CAD build for the part. Positions are in the model's coordinates, mm. A direction names the side the tool comes from. Give positions to 0.01 mm unless a question says otherwise; leave off trailing zeros. Write each loop counter-clockwise with the first axis right and the second up, starting at its lowest first coordinate (ties: lowest second). Pieces come first, ordered by that corner, then holes. Notation, with made-up numbers: (79, 18) - (105, 18) arc R15 cw to (105, 46) - close; hole circle Ø2 at (47, 79). An arc over 180 degrees is marked (long way). Put each result on its own line as item: value. Start each with the question number.
1. Wall check: line 1 (X direction, y = 1.7, z = 0); line 2 (Y direction, x = 0.9, z = 0); line 3 (Y direction, x = 1.3, z = 0). Give the ranges that are in metal, low to high.
2. Cut at B-B on z = 0. Give the number of separate pieces and of enclosed holes in the cut face, and give its area (3 significant figures).
3. Cut at A-A on x = 14.9. List the corners of the cut face in (y, z) (3 decimals).
4. Cut at D-D on x = 35. List the corners of the cut face in (y, z) (3 decimals), and give its area (3 significant figures).
5. Drop flat-ended pins along their axis: pin 1 (6 mm diameter, centred on x = 42.9, z = 0, fed in from -Y); pin 2 (8 mm diameter, centred on x = 18.5, z = 0, fed in from +Y) (3 decimals). Give the stop position or say it passes through.
6. Tool access for faces 5 (the flat face through (3.175, 28, 0)), 6 (the flat face through (14, 2, 7.9)): list every direction of +Z, -Z, +X, -X, +Y, -Y with a clear straight run to the whole face (end or side of a thin tool).
7. Cut at C-C on z = -5.25. List the corners of the cut face in (x, y) (3 decimals), and give its area (3 significant figures).
8. Mould opens along Y. For faces 1 (the cylindrical face through (1.1, 45.01, -1.34)), 2 (the cylindrical face through (1.1, 13.4, 2)), 3 (the flat face through (28, 0, 0)), 4 (the cylindrical face through (45.01, 1.1, 1.34)) say: +Y half, -Y half, draft (parallel to the pull), parting line (faces both ways), or undercut.
from build123d import *

# Parameters (mm, degrees)
FLANGE_BASE1_DEPTH    = 7.9
FILETE2_RADIUS        = 7.9
FILETE2_LENGTH        = 3.175
FILETE4_RADIUS        = 7.9
FILETE4_LENGTH        = 3.175
ESBO_O6_R             = 2.5
CORTE_EXTRUS_O1_DEPTH = 71.07988745
ESBO_O7_R             = 2.5
CORTE_EXTRUS_O2_DEPTH = 71.07988745
CHANFRO2_SIZE         = 1


# Sheet-metal steps are written as plain solids
with BuildPart() as part:
    # Esboço1 → Flange-base1 (new, symmetric)
    with BuildSketch(Plane.XY):
        with BuildLine():
            Line((50.8, 0), (4.175, 0))
            ThreePointArc((4.175, 0), (1.222829189, 1.222829189), (0, 4.175))
            Line((0, 4.175), (0, 50.8))
            Line((0, 50.8), (3.175, 50.8))
            Line((3.175, 50.8), (3.175, 4.175))
            ThreePointArc((3.175, 4.175), (3.467893219, 3.467893219), (4.175, 3.175))
            Line((4.175, 3.175), (50.8, 3.175))
            Line((50.8, 3.175), (50.8, 0))
        make_face()
    extrude(amount=FLANGE_BASE1_DEPTH, both=True)

    # Filete2: full round fillet: the end face becomes a half cylinder, R = half its width
    filete2_face = Plane((1.5875, 50.8, 0), x_dir=(1, 0, 0), z_dir=(0, 1, 0))  # on the end face: x along it, z out of the body
    filete2_slab = filete2_face.offset(-FILETE2_RADIUS / 2) * Box(FILETE2_LENGTH, 2 * FILETE2_RADIUS, FILETE2_RADIUS, mode=Mode.PRIVATE)  # the body's end, R deep
    filete2_round = Plane((1.5875, 42.9, 0), x_dir=(0, 1, 0), z_dir=(1, 0, 0)) * Cylinder(FILETE2_RADIUS, FILETE2_LENGTH, mode=Mode.PRIVATE)  # its axis R under the face
    add(filete2_slab - filete2_round, mode=Mode.SUBTRACT)

    # Filete4: full round fillet: the end face becomes a half cylinder, R = half its width
    filete4_face = Plane((50.8, 1.5875, 0), x_dir=(0, -1, 0), z_dir=(1, 0, 0))  # on the end face: x along it, z out of the body
    filete4_slab = filete4_face.offset(-FILETE4_RADIUS / 2) * Box(FILETE4_LENGTH, 2 * FILETE4_RADIUS, FILETE4_RADIUS, mode=Mode.PRIVATE)  # the body's end, R deep
    filete4_round = Plane((42.9, 1.5875, 0), x_dir=(1, 0, 0), z_dir=(0, -1, 0)) * Cylinder(FILETE4_RADIUS, FILETE4_LENGTH, mode=Mode.PRIVATE)  # its axis R under the face
    add(filete4_slab - filete4_round, mode=Mode.SUBTRACT)

    # Esboço6 → Corte-extrusão1 (cut, through all)
    with BuildSketch(Plane(origin=(0, 3.175, 0), x_dir=(1, 0, 0), z_dir=(0, 1, 0))):
        with Locations(Location((14.9, 0, 0), (0, 0, 270))):
            Circle(ESBO_O6_R)
        with Locations(Location((42.9, 0, 0), (0, 0, 270))):
            Circle(ESBO_O6_R)
    extrude(amount=-CORTE_EXTRUS_O1_DEPTH, mode=Mode.SUBTRACT)

    # Esboço7 → Corte-extrusão2 (cut, through all)
    with BuildSketch(Plane(origin=(3.175, 0, 0), x_dir=(0, 0, -1), z_dir=(1, 0, 0))):
        with Locations((0, 42.9)):
            Circle(ESBO_O7_R)
        with Locations((0, 14.9)):
            Circle(ESBO_O7_R)
    extrude(amount=-CORTE_EXTRUS_O2_DEPTH, mode=Mode.SUBTRACT)

    # Chanfro2
    chanfro2_edges = [part.edges().sort_by_distance(p)[0] for p in [
        (42.9, 3.175, -2.5),
        (14.9, 3.175, -2.5),
        (3.175, 42.9, 2.5),
        (3.175, 14.9, 2.5),
    ]]
    chamfer(chanfro2_edges, length=CHANFRO2_SIZE)


solid = part.part
Report:
1. line 1: x = 0.81 to 12.4, 17.4 to 40.4, 45.4 to 50.8
1. line 2: y = 1.59 to 12.4, 17.4 to 40.4, 45.4 to 50.8
1. line 3: y = 1.15 to 12.4, 17.4 to 40.4, 45.4 to 50.8
2. separate pieces: 5
2. enclosed holes: 0
2. area: 241 mm²
3. outline: (0, -7.9) - (3.175, -7.9) - (3.175, -3.5) - (2.175, -2.5) - (0, -2.5) - close; (0, 2.5) - (2.175, 2.5) - (3.175, 3.5) - (3.175, 7.9) - (0, 7.9) - close
4. outline: (0, -7.9) - (3.175, -7.9) - (3.175, 7.9) - (0, 7.9) - close
4. area: 50.2 mm²
5. pin 1: stops at y = 0
5. pin 2: stops at y = 3.175
6. face 5: +Z, -Z, +X, +Y
6. face 6: +Z, +X, -X, +Y, -Y
7. outline: (0, 4.175) arc R4.175 ccw to (4.175, 0) - (48.803, 0) - (48.803, 3.175) - (4.175, 3.175) arc R1 cw to (3.175, 4.175) - (3.175, 48.803) - (0, 48.803) - close
7. area: 296 mm²
8. face 1: undercut
8. face 2: undercut
8. face 3: -Y half
8. face 4: draft
